Verification items for the finished model (mm, model axes). Give positions to 0.01 mm unless a question says otherwise; leave off trailing zeros. Write each loop counter-clockwise with the first axis right and the second up, starting at its lowest first coordinate (ties: lowest second). Pieces come first, ordered by that corner, then holes.
Autodesk Inventor part; units mm, degrees
ref_plane "YZ Plane" through (0, 0, 0) normal (1, 0, 0) x (0, 1, 0)
ref_plane "XZ Plane" through (0, 0, 0) normal (0, 1, 0) x (-1, 0, 0)
ref_plane "XY Plane" through (0, 0, 0) normal (0, 0, 1) x (1, 0, 0)
sketch "Szkic1" plane through (0, 0, 0) normal (0, 0, 1) x (1, 0, 0)
  line L0 (-10.326, 7.3757) -> (12.674, 7.3757)
  line L1 (12.674, 7.3757) -> (12.674, -8.1243)
  line L2 (12.674, -8.1243) -> (-10.326, -8.1243)
  line L3 (-10.326, -8.1243) -> (-10.326, 7.3757)
  point P0 (0, 0)
  point P1 (-6.326, -0.3743)
  point P2 (8.674, -0.3743)
  dimension "d0" = 23
  dimension "d1" = 15.5
  dimension "d4" = 7.75
  dimension "d5" = 7.75
  dimension "d6" = 4
  dimension "d7" = 4
extrude "Wyciągnięcie proste1" add sketch "Szkic1" along normal blind 3
hole "Otwór1" at (-6.326, -0.3743, 0) at (8.674, -0.3743, 0) direction (0, 0, 1) diameter 3 end through all
chamfer "Faza1" distance 1.5 angle 45 4 edges at (12.674, -8.1243, 1.5) (-10.326, -8.1243, 1.5) (-10.326, 7.3757, 1.5) (12.674, 7.3757, 1.5)
properties part number "LC_ALU_3mm_Timing_Belt_Clamp_Y_Axis"
Item 1: Sectioned sample at D-D on y = 6.5. Record the cut outline in (x, z).
Answer key:
outline: (-9.7, 0) - (12.05, 0) - (12.05, 3) - (-9.7, 3) - close
Item 2: Sectioned sample at A-A on x = -6. Record the cut outline in (y, z), then the cut area to 3 significant figures.
Answer key:
outline: (-8.12, 0) - (-1.84, 0) - (-1.84, 3) - (-8.12, 3) - close; (1.09, 0) - (7.38, 0) - (7.38, 3) - (1.09, 3) - close
area: 37.7 mm2
Item 3: Sectioned sample at B-B on y = -0.25. Record the cut outline in (x, z).
Answer key:
outline: (-10.33, 0) - (-7.82, 0) - (-7.82, 3) - (-10.33, 3) - close; (-4.83, 0) - (7.18, 0) - (7.18, 3) - (-4.83, 3) - close; (10.17, 0) - (12.67, 0) - (12.67, 3) - (10.17, 3) - close
Item 4: Sectioned sample at C-C on z = 1.15. Record the cut outline in (x, y), then the cut area to 3 significant figures.
Answer key:
outline: (-10.33, -6.62) - (-8.83, -8.12) - (11.17, -8.12) - (12.67, -6.62) - (12.67, 5.88) - (11.17, 7.38) - (-8.83, 7.38) - (-10.33, 5.88) - close; hole circle Ø3 at (-6.33, -0.37); hole circle Ø3 at (8.67, -0.37)
area: 338 mm2
Item 5: Release check for a two-part mould opening along Y. For faces 1 (the face through (7.187, -0.57, 1.521)), 2 (the face through (-10.326, 0, 1)), 3 (the face through (1, -8.124, 1)) record: released by +Y, released by -Y, zero draft, split by the parting line, or undercut.
Answer key:
face 1: undercut
face 2: zero draft
face 3: released by -Y
Item 6: Scan lines: line 1 along X through (y, z) = (-1.25, 1.7); line 2 along X through (y, z) = (1, 2.25); line 3 along X through (y, z) = (-6.75, 0.45). Record each from-to range of solid material in increasing order.
Answer key:
line 1: x = -10.33 to -7.54, -5.11 to 7.46, 9.89 to 12.67
line 2: x = -10.33 to -6.93, -5.72 to 8.07, 9.28 to 12.67
line 3: x = -10.2 to 12.55
Item 7: Depth check by flat-ended pin: pin 1 (1.8 mm diameter, centred on x = -6.33, y = -0.37, fed in from +Z). Enter the tip coordinate at first touch or a pass-through.
Answer key:
pin 1: passes through
